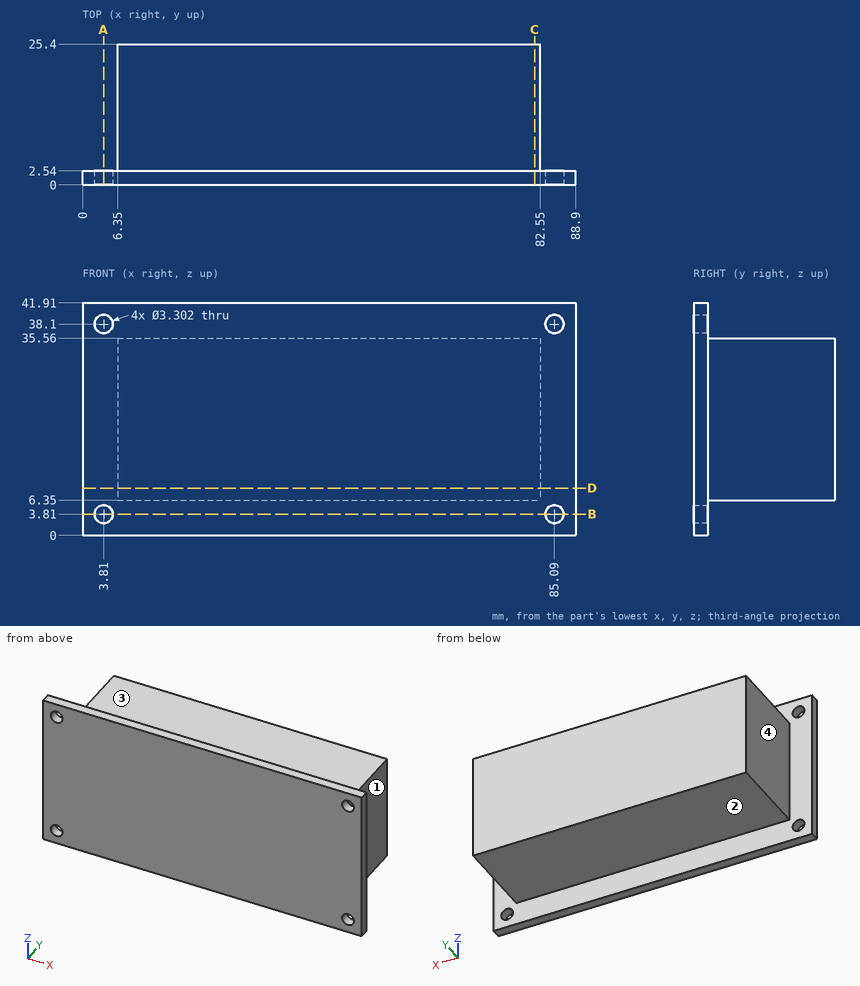
Verification items for this drawing (mm, ordinates from the low corner). A direction names the side the tool comes from. Round coordinates to 2 decimals unless told otherwise and drop trailing zeros. Order: outer loops, then holes, each group sorted by start corner. A loop starts at its lowest first (then second) coordinate and runs counter-clockwise, first axis right, second up. Notation, with made-up numbers: (43.5, -37.5) - (48.5, -37.5) arc R19 ccw to (48.5, -32.5) - close; hole circle Ø10 at (-27.5, -18). An arc over 180 degrees is marked (long way). Use CSV: the item, a comma, the result in double quotes.
(1) Section check C-C on x = 81.5. Record the boundary of the cut face in (y, z).
Entries:
outline,"(0, 0) - (2.54, 0) - (2.54, 6.35) - (25.4, 6.35) - (25.4, 35.56) - (2.54, 35.56) - (2.54, 41.91) - (0, 41.91) - close"
(2) Thickness scan on probe 1 along Z at (x, y) = (85.09, 0.7); probe 2 along X at (y, z) = (0.65, 3.81); probe 3 along X at (y, z) = (9.5, 33). Record the ranges inside material, lowest first. Write a range as from..to.
Entries:
probe 1,"0..2.16, 5.46..36.45, 39.75..41.91"
probe 2,"0..2.16, 5.46..83.44, 86.74..88.9"
probe 3,"6.35..82.55"
(3) Access from +Z, -Z, +X, -X, +Y, -Y to the whole of each face (thin tool, end or side, straight path). Record for the marked faces 1, 2, 3 and 4.
Entries:
face 1,"+Z, -Z, +X, +Y"
face 2,"-Z, +X, -X, +Y"
face 3,"+Z, +X, -X, +Y"
face 4,"+Z, -Z, -X, +Y"
(4) Gauge pin test, flat ends, axial feed: pin 1 Ø12 at (x, y) = (65.5, 15.5) entering from +Z; pin 2 Ø10 at (y, z) = (3, 6) entering from -X; pin 3 Ø1.5 at (y, z) = (7, 13) entering from +X; pin 4 Ø3 at (x, z) = (85.09, 38.1) entering from +Y. Record the tip position at first contact, or that the pin passes through.
Entries:
pin 1,"z = 35.56"
pin 2,"x = 0"
pin 3,"x = 82.55"
pin 4,"through"
(5) Section check D-D on z = 8.5. Record the boundary of the cut face in (x, y), and give its area (3 significant figures).
Entries:
outline,"(0, 0) - (88.9, 0) - (88.9, 2.54) - (82.55, 2.54) - (82.55, 25.4) - (6.35, 25.4) - (6.35, 2.54) - (0, 2.54) - close"
area,"1,970 mm^2"
(6) Section check A-A on x = 3.81. Record the boundary of the cut face in (y, z), and give its area (3 significant figures).
Entries:
outline,"(0, 0) - (2.54, 0) - (2.54, 2.16) - (0, 2.16) - close; (0, 5.46) - (2.54, 5.46) - (2.54, 36.45) - (0, 36.45) - close; (0, 39.75) - (2.54, 39.75) - (2.54, 41.91) - (0, 41.91) - close"
area,"89.7 mm^2"
(7) Section check B-B on z = 3.81. Record the boundary of the cut face in (x, y), and give its area (3 significant figures).
Entries:
outline,"(0, 0) - (2.16, 0) - (2.16, 2.54) - (0, 2.54) - close; (5.46, 0) - (83.44, 0) - (83.44, 2.54) - (5.46, 2.54) - close; (86.74, 0) - (88.9, 0) - (88.9, 2.54) - (86.74, 2.54) - close"
area,"209 mm^2"
